The figure shows three views and two pictorial views of one solid part (mm, origin at its lowest corner). Answer the questions. Coordinates: 2 decimals unless noted, no trailing zeros. Loops run counter-clockwise (first coordinate to the right, second up) from the corner with the lowest first, then second, coordinate; pieces in that order, holes last. Notation, with made-up numbers: (-13.5, 8.5) -> (34.5, 8.5) arc R24 ccw to (34.5, 45.5) -> close; hole circle Ø8 at (43, 45.5). An arc over 180 degrees is marked (long way). Answer as a JSON object with one key per item and string values. Group by question number.
1) Section B-B, the plane z = 11.5 is taken. Give the vertices of the cut face in (x, y).
2) Flat-ended cylindrical pins translate along their axes: P1, Ø8, axis at x = 79, z = 52.5, coming from the +Y side; P2, Ø1, axis at x = 60, y = 2.5, coming from the +Z side; P3, Ø1, axis at x = 73.5, y = 3, coming from the +Z side (1 decimal); P4, Ø1.5, axis at x = 29.5, y = 2, coming from the -Z side (1 decimal). Find the tip coordinate at first contact, or state that the pin passes through.
3) Consider probe 1 along Z at (x, y) = (47, 1.55); probe 2 along X at (y, z) = (0.45, 17.5) (1 decimal); probe 3 along Z at (x, y) = (76, 0.4) (1 decimal). Determine where each line is inside the solid, lowest interval first. Write a range as [from, to].
4) Section D-D, the plane y = 2.9 is taken. Count the separate pieces of the cut face and the enclosed holes in it, plus the area to 3 significant figures.
5) Section C-C, the plane x = 5 is taken. Give the vertices of the cut face in (y, z) (1 decimal).
6) Section A-A, the plane z = 47 is taken. Give the vertices of the cut face in (x, y), plus the area to 3 significant figures.
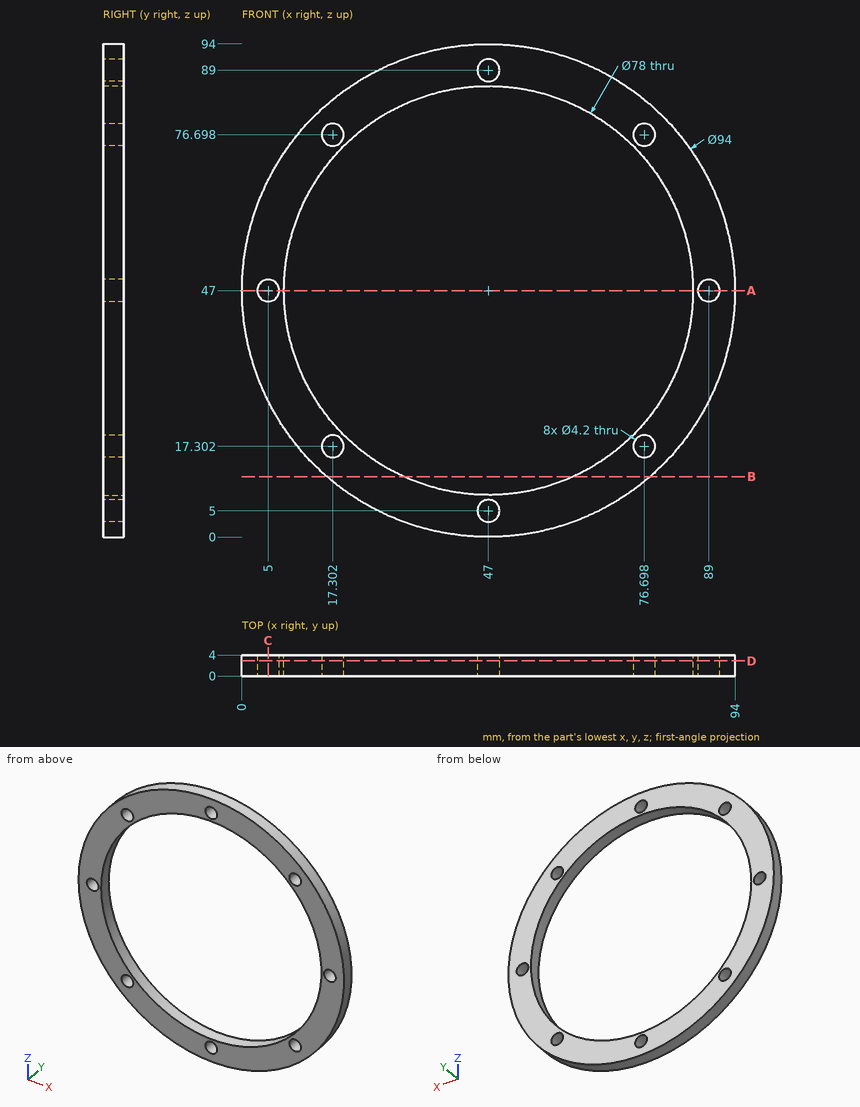
Determined:
{
 "1": {"outline": "(16.2, 0) -> (30.85, 0) -> (30.85, 4) -> (16.2, 4) -> close; (63.15, 0) -> (77.8, 0) -> (77.8, 4) -> (63.15, 4) -> close"},
 "2": {"P1": "through", "P2": "z = 92.31", "P3": "z = 86.2", "P4": "z = 3.1"},
 "3": {"probe 1": "[0, 2.9], [7.1, 8], [86, 86.9], [91.1, 94]", "probe 2": "[10.4, 15.2], [19.4, 21.5], [72.5, 74.6], [78.8, 83.6]", "probe 3": "[10, 15.3], [19.3, 20.9], [73.1, 74.7], [78.7, 84]"},
 "4": {"separate pieces": "1", "enclosed holes": "9", "area": "2,050 mm²"},
 "5": {"outline": "(0, 25.9) -> (4, 25.9) -> (4, 44.9) -> (0, 44.9) -> close; (0, 49.1) -> (4, 49.1) -> (4, 68.1) -> (0, 68.1) -> close"},
 "6": {"outline": "(0, 0) -> (2.9, 0) -> (2.9, 4) -> (0, 4) -> close; (7.1, 0) -> (8, 0) -> (8, 4) -> (7.1, 4) -> close; (86, 0) -> (86.9, 0) -> (86.9, 4) -> (86, 4) -> close; (91.1, 0) -> (94, 0) -> (94, 4) -> (91.1, 4) -> close", "area": "30.4 mm²"}
}
